```python
from build123d import *

# Parameters (mm, degrees)
F0_W     = 152.4
F0_H     = 76.2
F1_DEPTH = 101.6
F2_R     = 12.5
F3_DEPTH = 91.44
F4_W     = 5.08
F4_H     = 5.08
F5_DEPTH = 5.08


with BuildPart() as f1:
    # F0 (on Top) → F1 (new body)
    with BuildSketch(Plane.XY):
        with Locations((-332.398888, 3.914099)):
            Rectangle(F0_W, F0_H)
    extrude(amount=F1_DEPTH)

    # F2 (on face) → F3 (cut)
    with BuildSketch(Plane.XY.offset(101.6)):
        with Locations((-393.698888, 19.354099)):
            Circle(F2_R)
        with Locations((-353.698888, 19.354099)):
            Circle(F2_R)
        with Locations((-313.698888, 19.354099)):
            Circle(F2_R)
        with Locations((-273.698888, -11.525901)):
            Circle(F2_R)
        with Locations((-313.698888, -11.525901)):
            Circle(F2_R)
        with Locations((-353.698888, -11.525901)):
            Circle(F2_R)
        with Locations((-393.698888, -11.525901)):
            Circle(F2_R)
        with Locations((-273.698888, 19.354099)):
            Circle(F2_R)
    extrude(amount=-F3_DEPTH, mode=Mode.SUBTRACT)

    # F4 (on face) → F5 (join)
    with BuildSketch(Plane(origin=(0, 0, 0), x_dir=(1, 0, 0), z_dir=(0, 0, -1))):
        with Locations((-403.518888, 29.105901)):
            Rectangle(F4_W, F4_H)
        with Locations((-403.518888, -36.934099)):
            Rectangle(F4_W, F4_H)
        with Locations((-261.278888, -36.934099)):
            Rectangle(F4_W, F4_H)
        with Locations((-261.278888, 29.105901)):
            Rectangle(F4_W, F4_H)
    extrude(amount=F5_DEPTH)


solid = f1.part
```
Input: part model. Units: mm. Frame: model coordinates. A direction names the side the tool comes from. Round coordinates to 2 decimals unless told otherwise and drop trailing zeros. Loops run counter-clockwise (first coordinate to the right, second up) from the corner with the lowest first, then second, coordinate; pieces in that order, holes last. Notation, with made-up numbers: (-18.5, 37) - (18.5, 37) arc R17 ccw to (18.5, 67) - close; hole circle Ø9 at (-8, 32). An arc over 180 degrees is marked (long way). One line per item, written item: value. Start each with the question number.
(1) Draft query along Y for faces 1 (the flat face through (-408.599, 3, 50)), 2 (the flat face through (-354, -11, 10.16)), 3 (the flat face through (-333, 42.014, 50)). Return one class per face: +Y half, -Y half, draft (parallel to the pull), parting line (faces both ways), or undercut.
(2) Section C-C, the plane y = 14. Return loops of the section in (x, z).
(3) Contact query for flat-ended pins moving along their axis: P1, Ø5.5, axis at x = -261, z = -3.5, coming from the +Y side; P2, Ø5, axis at x = -315.5, y = -16, coming from the -Z side; P3, Ø5.5, axis at y = -29, z = -4, coming from the -X side. Output: stop coordinate, or through.
(4) Section A-A, the plane z = 38. Count the separate pieces of the cut face and the enclosed holes in it, plus the area to 3 significant figures.
(5) Section D-D, the plane x = -266.5. Return loops of the section in (y, z).
(6) Ray query, line 1 (X direction, y = -7, z = 66.5); line 2 (Y direction, x = -313, z = 11); line 3 (Y direction, x = -305.5, z = 24). Return the intervals inside material, ascending. Write a range as [from, to].
(7) Section B-B, the plane x = -385. Return loops of the section in (y, z).
(8) Access query for faces 4 (the cylindrical face through (-326.187, 19.904, 56.52)), 5 (the flat face through (-406.059, -29, -3)), 6 (the flat face through (-404, -26.566, -3)), 7 (the flat face through (-400.979, -29, -3)). Directions: +Z, -Z, +X, -X, +Y, -Y. A direction counts if a zero-diameter tool reaches every point of the face in a straight line with its end or side. Return the directions, or none.
Results below:
1. face 1: draft
1. face 2: undercut
1. face 3: +Y half
2. outline: (-408.6, 0) - (-256.2, 0) - (-256.2, 101.6) - (-262.4, 101.6) - (-262.4, 10.16) - (-284.99, 10.16) - (-284.99, 101.6) - (-302.4, 101.6) - (-302.4, 10.16) - (-324.99, 10.16) - (-324.99, 101.6) - (-342.4, 101.6) - (-342.4, 10.16) - (-364.99, 10.16) - (-364.99, 101.6) - (-382.4, 101.6) - (-382.4, 10.16) - (-404.99, 10.16) - (-404.99, 101.6) - (-408.6, 101.6) - close
3. P1: y = 39.47
3. P2: z = 0
3. P3: x = -406.06
4. separate pieces: 1
4. enclosed holes: 8
4. area: 7,690 mm^2
5. outline: (-34.19, 0) - (42.01, 0) - (42.01, 101.6) - (29.57, 101.6) - (29.57, 10.16) - (9.14, 10.16) - (9.14, 101.6) - (-1.31, 101.6) - (-1.31, 10.16) - (-21.74, 10.16) - (-21.74, 101.6) - (-34.19, 101.6) - close
6. line 1: [-408.6, -405.35], [-382.05, -365.35], [-342.05, -325.35], [-302.05, -285.35], [-262.05, -256.2]
6. line 2: [-34.19, -24.01], [0.95, 6.87], [31.83, 42.01]
6. line 3: [-34.19, -20.96], [-2.09, 9.92], [28.79, 42.01]
7. outline: (-34.19, 0) - (42.01, 0) - (42.01, 101.6) - (28.33, 101.6) - (28.33, 10.16) - (10.38, 10.16) - (10.38, 101.6) - (-2.55, 101.6) - (-2.55, 10.16) - (-20.5, 10.16) - (-20.5, 101.6) - (-34.19, 101.6) - close
8. face 4: +Z
8. face 5: -Z, -X, +Y, -Y
8. face 6: -Z, +X, -X
8. face 7: -Z, +Y, -Y
